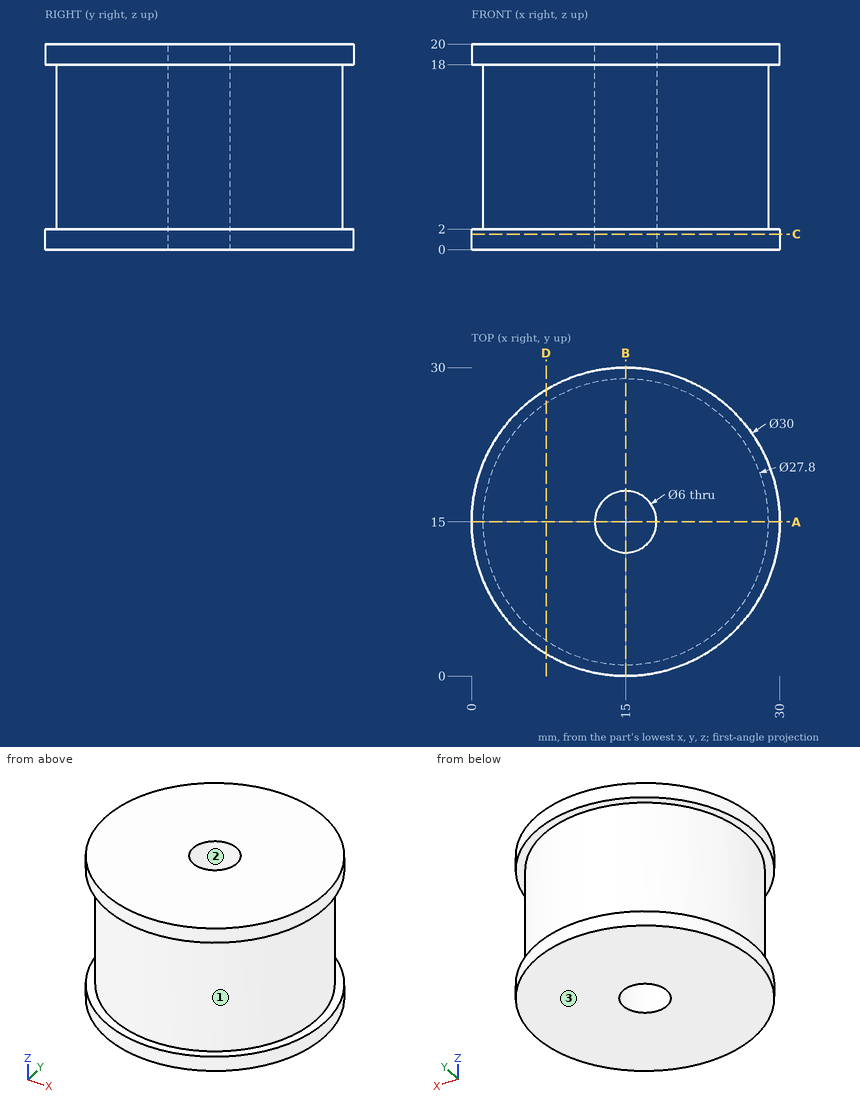
Geometry check sheet. Reference: drawing and pictorial views, mm from the part's lowest x, y, z. Round coordinates to 2 decimals unless told otherwise and drop trailing zeros. Loops run counter-clockwise (first coordinate to the right, second up) from the corner with the lowest first, then second, coordinate; pieces in that order, holes last. Notation, with made-up numbers: (0.25, -3) - (37.25, -3) arc R20 cw to (37.25, 6) - close; hole circle Ø3 at (61, 29.25). An arc over 180 degrees is marked (long way). One line per question, with ' | ' between items. Start each with the question number.
1. Cross-section at A-A on y = 15. Record the cut outline in (x, z).
2. Cross-section at C-C on z = 1.5. Record the cut outline in (x, y), then the cut area to 3 significant figures.
3. Draft check along Y on the marked faces 1, 2 and 3. Enter one of: released by +Y, released by -Y, zero draft, split by the parting line, or undercut.
4. Scan lines: line 1 (Z direction, x = 25.25, y = 4.75); line 2 (Y direction, x = 15, z = 11.75); line 3 (X direction, y = 19, z = 3.5). Record each from-to range of solid material in increasing order. Write a range as [from, to].
5. Depth check by flat-ended pin: pin 1 (8 mm diameter, centred on x = 11, y = 10, fed in from -Z); pin 2 (10 mm diameter, centred on x = 26, z = 7, fed in from +Y); pin 3 (4 mm diameter, centred on x = 17.5, z = 12, fed in from -Y); pin 4 (8 mm diameter, centred on y = 22.5, z = 15.5, fed in from +X). Enter the tip coordinate at first touch or a pass-through.
6. Cross-section at D-D on x = 7.25. Record the cut outline in (y, z).
Taken from the geometry:
1) outline: (0, 0) - (12, 0) - (12, 20) - (0, 20) - (0, 18) - (1.1, 18) - (1.1, 2) - (0, 2) - close; (18, 0) - (30, 0) - (30, 2) - (28.9, 2) - (28.9, 18) - (30, 18) - (30, 20) - (18, 20) - close
2) outline: circle Ø30 at (15, 15); hole circle Ø6 at (15, 15) | area: 679 mm²
3) face 1: split by the parting line | face 2: undercut | face 3: zero draft
4) line 1: [0, 2], [18, 20] | line 2: [1.1, 12], [18, 28.9] | line 3: [1.69, 28.31]
5) pin 1: z = 0 | pin 2: y = 27.54 | pin 3: y = 1.11 | pin 4: x = 29.35
6) outline: (2.16, 0) - (27.84, 0) - (27.84, 2) - (26.54, 2) - (26.54, 18) - (27.84, 18) - (27.84, 20) - (2.16, 20) - (2.16, 18) - (3.46, 18) - (3.46, 2) - (2.16, 2) - close
